from build123d import *

# Parameters (mm, degrees)
F0_W     = 124.5
F0_H     = 36.4
F0_R     = 2.46
F0_W_2   = 51.32
F0_H_2   = 6.6
F0_W_3   = 51.308
F1_DEPTH = 6
F2_R     = 3.3
F3_R     = 3.29999
F4_R     = 3.3
F5_R     = 3.29999
F6_R     = 3.3
F7_R     = 3.29999
F8_R     = 3.3
F9_R     = 3.29999


# Not quite as in the source:
# - a fillet or chamfer is up to 0.001 mm smaller than in the source, because OpenCascade refuses the exact size


with BuildPart() as f1:
    # F0 (on Front) → F1 (new body)
    with BuildSketch(Plane.XZ):
        Rectangle(F0_W, F0_H)
        with Locations((-56.75, -10)):
            Circle(F0_R, mode=Mode.SUBTRACT)
        with Locations((-27.16, 0)):
            Rectangle(F0_W_2, F0_H_2, mode=Mode.SUBTRACT)
        with Locations((56.75, -10)):
            Circle(F0_R, mode=Mode.SUBTRACT)
        with Locations((27.154, 0)):
            Rectangle(F0_W_3, F0_H_2, mode=Mode.SUBTRACT)
        with Locations((-57.25, 10)):
            Circle(F0_R, mode=Mode.SUBTRACT)
        with Locations((56.75, 10)):
            Circle(F0_R, mode=Mode.SUBTRACT)
    extrude(amount=F1_DEPTH)

    # F2
    f2_edges = [f1.edges().sort_by_distance(p)[0] for p in [
        (-52.82, -3, -3.3),
    ]]
    fillet(f2_edges, radius=F2_R)

    # F3 (radius 3.3 in the source; OpenCascade refuses exactly that, so slightly less here)
    f3_edges = [f1.edges().sort_by_distance(p)[0] for p in [
        (-52.82, -3, 3.3),
    ]]
    fillet(f3_edges, radius=F3_R)

    # F4
    f4_edges = [f1.edges().sort_by_distance(p)[0] for p in [
        (-1.5, -3, 3.3),
    ]]
    fillet(f4_edges, radius=F4_R)

    # F5 (radius 3.3 in the source; OpenCascade refuses exactly that, so slightly less here)
    f5_edges = [f1.edges().sort_by_distance(p)[0] for p in [
        (-1.5, -3, -3.3),
    ]]
    fillet(f5_edges, radius=F5_R)

    # F6
    f6_edges = [f1.edges().sort_by_distance(p)[0] for p in [
        (1.5, -3, 3.3),
    ]]
    fillet(f6_edges, radius=F6_R)

    # F7 (radius 3.3 in the source; OpenCascade refuses exactly that, so slightly less here)
    f7_edges = [f1.edges().sort_by_distance(p)[0] for p in [
        (1.5, -3, -3.3),
    ]]
    fillet(f7_edges, radius=F7_R)

    # F8
    f8_edges = [f1.edges().sort_by_distance(p)[0] for p in [
        (52.808, -3, 3.3),
    ]]
    fillet(f8_edges, radius=F8_R)

    # F9 (radius 3.3 in the source; OpenCascade refuses exactly that, so slightly less here)
    f9_edges = [f1.edges().sort_by_distance(p)[0] for p in [
        (52.808, -3, -3.3),
    ]]
    fillet(f9_edges, radius=F9_R)


solid = f1.part
Here's how the part is built. I have some questions about the finished solid (model axes, mm). A direction names the side the tool comes from. Round coordinates to 2 decimals unless told otherwise and drop trailing zeros. Order: outer loops, then holes, each group sorted by start corner. A loop starts at its lowest first (then second) coordinate and runs counter-clockwise, first axis right, second up. Notation, with made-up numbers: M 14.25,64.25 L 24.25,64.25 A27 cw 24.25,85.25 Z; hole C -3,-20 d3. An arc over 180 degrees is marked long. Return JSON: item names as keys, results as strings. Group by question number.
1. If we mould it in two halves opening along Z, with no side actions, what happens to faces 3 (the face through (62.25, -3, 0)), 4 (the face through (-27, -3, 3.3)), 5 (the face through (-1, -3, -18.2)), 6 (the face through (-2.492, -3.042, 2.359))? For each: pulls with the +Z half, pulls with the -Z half, needs draft (parallel to the pull), parting line crosses it, or undercut.
2. If we section it at B-B on z = 10: List the corners of the cut face in (x, y) for me, then the cut area to 3 significant figures.
3. I'm going to push a flat-ended pin straight in: pin 1 Ø4 at (x, z) = (45.5, -7.5) entering from +Y. Where does the tip first touch, or does it pass through?
4. If we section it at A-A on x = 56.75: List the corners of the cut face in (y, z) for me, then the cut area to 3 significant figures.
5. Please list where these lines run through material, in increasing order: probe 1 along Z at (x, y) = (56.75, -2.85); probe 2 along Z at (x, y) = (-18, -2.1); probe 3 along Z at (x, y) = (-57.25, -2.3).
6. If we section it at C-C on y = -4.7: State how many separate pieces and enclosed holes the cut face has, then the cut area to 3 significant figures.
7. On a 3-axis mill with a long thin cutter (end or side, diameter ignored), from which of +Z, -Z, +X, -X, +Y, -Y can I reach the whole of each face in a straight line? I mean faces 1 (the face through (51.867, -3.042, -2.308)), 2 (the face through (-1, 0, 0)). Say none if no direction works.
Reply:
{
 "1": {"face 3": "needs draft", "face 4": "undercut", "face 5": "pulls with the -Z half", "face 6": "undercut"},
 "2": {"outline": "M -62.25,-6 L -59.71,-6 L -59.71,0 L -62.25,0 Z; M -54.79,-6 L 54.29,-6 L 54.29,0 L -54.79,0 Z; M 59.21,-6 L 62.25,-6 L 62.25,0 L 59.21,0 Z", "area": "688 mm^2"},
 "3": {"pin 1": "y = 0"},
 "4": {"outline": "M -6,-18.2 L 0,-18.2 L 0,-12.46 L -6,-12.46 Z; M -6,-7.54 L 0,-7.54 L 0,7.54 L -6,7.54 Z; M -6,12.46 L 0,12.46 L 0,18.2 L -6,18.2 Z", "area": "159 mm^2"},
 "5": {"probe 1": "-18.2 to -12.46, -7.54 to 7.54, 12.46 to 18.2", "probe 2": "-18.2 to -3.3, 3.3 to 18.2", "probe 3": "-18.2 to -12.41, -7.59 to 7.54, 12.46 to 18.2"},
 "6": {"separate pieces": "1", "enclosed holes": "6", "area": "3,800 mm^2"},
 "7": {"face 1": "+Y, -Y", "face 2": "+Z, -Z, +X, -X, +Y"}
}
